```python
from build123d import *

# Parameters (mm, degrees)
SKETCH_1_R          = 7.6
SKETCH_1_R_2        = 5.2
EXTRUDE_1_DEPTH     = 120
SKETCH_2_R          = 20
EXTRUDE_2_DEPTH     = 20
CUT_EXTRUDE_START   = -157
SKETCH_3_R          = 5.2
CUT_EXTRUDE_1_DEPTH = 157
FILLET_1_R          = 5
FILLET_2_R          = 2
FILLET_3_R          = 1


with BuildPart() as part:
    # 草图1 → 凸台-拉伸1 (new body)
    with BuildSketch(Plane(origin=(0, 0, 0), x_dir=(1, 0, 0), z_dir=(0, 1, 0))):
        with Locations(Location((0, 0, 0), (0, 0, 270))):
            Circle(SKETCH_1_R)
        with Locations(Location((0, 0, 0), (0, 0, 270))):
            Circle(SKETCH_1_R_2, mode=Mode.SUBTRACT)
    extrude(amount=EXTRUDE_1_DEPTH)

    # 草图2 → 凸台-拉伸2 (add)
    with BuildSketch(Plane(origin=(0, 120, 0), x_dir=(1, 0, 0), z_dir=(0, 1, 0))):
        with Locations(Location((0, 0, 0), (0, 0, 270))):
            Circle(SKETCH_2_R)
    extrude(amount=EXTRUDE_2_DEPTH)

    # 草图3 → 切除-拉伸1 (cut)
    with BuildSketch(Plane(origin=(0, 140, 0), x_dir=(1, 0, 0), z_dir=(0, 1, 0)).offset(CUT_EXTRUDE_START)):
        with Locations(Location((0, 0, 0), (0, 0, 270))):
            Circle(SKETCH_3_R)
    extrude(amount=CUT_EXTRUDE_1_DEPTH, mode=Mode.SUBTRACT)

    # 圆角1
    fillet_1_edges = [part.edges().sort_by_distance(p)[0] for p in [
        (0, 140, -20),
        (0, 120, -20),
    ]]
    fillet(fillet_1_edges, radius=FILLET_1_R)

    # 圆角2
    fillet_2_edges = [part.edges().sort_by_distance(p)[0] for p in [
        (0, 0, -7.6),
        (0, 120, -7.6),
    ]]
    fillet(fillet_2_edges, radius=FILLET_2_R)

    # 圆角3
    fillet_3_edges = [part.edges().sort_by_distance(p)[0] for p in [
        (0, 140, -5.2),
    ]]
    fillet(fillet_3_edges, radius=FILLET_3_R)


solid = part.part
```
Check sheet for the modelled part. Datum: model origin and axes. Units: mm. Give positions to 0.01 mm unless a question says otherwise; leave off trailing zeros. Write each loop counter-clockwise with the first axis right and the second up, starting at its lowest first coordinate (ties: lowest second). Pieces come first, ordered by that corner, then holes. Notation, with made-up numbers: (5.25, -38) - (49.25, -38) arc R13 cw to (49.25, -18) - close; hole circle Ø9 at (36.25, -5.75). An arc over 180 degrees is marked (long way). Answer as a JSON object with one key per item and string values. Group by question number.
1) Release check for a two-part mould opening along X. For faces 1 (the face through (0, 120, 10)), 2 (the face through (1.56, 68.53, 4.96)), 3 (the face through (-2.91, 59.19, 7.02)) record: pulls with the +X half, pulls with the -X half, needs draft (parallel to the pull), parting line crosses it, or undercut.
2) Sectioned sample at C-C (y = 103.5). Record the cut outline in (x, z), then the cut area to 3 significant figures.
3) Thickness scan on probe 1 along X at (y, z) = (31, 0); probe 2 along Y at (x, z) = (-13.5, -6.5); probe 3 along X at (y, z) = (72, 3). Record the ranges inside material, lowest first. Write a range as from..to.
4) Sectioned sample at A-A (x = 0). Record the cut outline in (y, z).
5) Sectioned sample at B-B (z = 0). Record the cut outline in (x, y).
6) Depth check by flat-ended pin: P1, Ø5, axis at x = 5, y = 115, coming from the -Z side; P2, Ø16.5, axis at x = 0, z = 0, coming from the -Y side; P3, Ø1.5, axis at x = 7.5, y = 76, coming from the +Z side. Enter the tip coordinate at first touch or a pass-through.
Geometry results:
{
 "1": {"face 1": "needs draft", "face 2": "undercut", "face 3": "parting line crosses it"},
 "2": {"outline": "circle Ø15.2 at (0, 0); hole circle Ø10.4 at (0, 0)", "area": "96.5 mm^2"},
 "3": {"probe 1": "x = -7.6..-5.2, 5.2..7.6", "probe 2": "y = 120..140", "probe 3": "x = -6.98..-4.25, 4.25..6.98"},
 "4": {"outline": "(0, -5.6) arc R2 ccw to (2, -7.6) - (118, -7.6) arc R2 cw to (120, -9.6) - (120, -15) arc R5 ccw to (125, -20) - (135, -20) arc R5 ccw to (140, -15) - (140, -6.2) arc R1 ccw to (139, -5.2) - (0, -5.2) - close; (0, 5.2) - (139, 5.2) arc R1 ccw to (140, 6.2) - (140, 15) arc R5 ccw to (135, 20) - (125, 20) arc R5 ccw to (120, 15) - (120, 9.6) arc R2 cw to (118, 7.6) - (2, 7.6) arc R2 ccw to (0, 5.6) - close"},
 "5": {"outline": "(-20, 125) arc R5 ccw to (-15, 120) - (-9.6, 120) arc R2 cw to (-7.6, 118) - (-7.6, 2) arc R2 ccw to (-5.6, 0) - (-5.2, 0) - (-5.2, 139) arc R1 ccw to (-6.2, 140) - (-15, 140) arc R5 ccw to (-20, 135) - close; (5.2, 0) - (5.6, 0) arc R2 ccw to (7.6, 2) - (7.6, 118) arc R2 cw to (9.6, 120) - (15, 120) arc R5 ccw to (20, 125) - (20, 135) arc R5 ccw to (15, 140) - (6.2, 140) arc R1 ccw to (5.2, 139) - close"},
 "6": {"P1": "stops at z = -7.18", "P2": "stops at y = 0", "P3": "stops at z = 3.49"}
}
